from build123d import *

# Parameters (mm, degrees)
SKETCH_1_R          = 1.7
SKETCH_1_R_2        = 4
EXTRUDE_1_DEPTH     = 2
SKETCH_2_R          = 1.5
SKETCH_2_R_2        = 1.7
SKETCH_2_R_3        = 1.65
CUT_EXTRUDE_2_DEPTH = 100.30986231


with BuildPart() as part:
    # Эскиз1 → Бобышка-Вытянуть1 (new body)
    with BuildSketch(Plane(origin=(0, 0, 0), x_dir=(1, 0, 0), z_dir=(0, 1, 0))):
        with BuildLine():
            Line((-11.994516295, 0.362737998), (-27.997650279, 0.362737998))
            ThreePointArc((-27.997650279, 0.362737998), (-19.670324553, 19.926824433), (0, 28))
            ThreePointArc((0, 28), (10.092907112, 26.117680334), (18.828808684, 20.72380186))
            Line((18.828808684, 20.72380186), (46.640586318, -4.544855106))
            add(Edge.make_bspline(
                [(73.991805315, -64.992405718), (82.088977067, -40.455490793), (46.640586318, -4.544855106)],
                knots=[0.235504237, 0.235504237, 0.235504237, 1.570796327, 1.570796327, 1.570796327], degree=2, weights=[1, 0.785281266, 1]))
            Line((73.991805315, -64.992405718), (67.937451343, -58.859103325))
            add(Edge.make_bspline(
                [(67.937451343, -58.859103325), (68.070075227, -1.227091326), (11.741792344, -2.475946799)],
                knots=[3.541017893, 3.541017893, 3.541017893, 5.906750707, 5.906750707, 5.906750707], degree=2, weights=[1, 0.378272966, 1]))
            ThreePointArc((11.741792344, -2.475946799), (-1.424956207, -11.915095459), (-11.994516295, 0.362737998))
        make_face()
        with Locations(Location((-6.322604321, 6.40505071, 0), (0, 0, 270))):
            Circle(SKETCH_1_R, mode=Mode.SUBTRACT)
        with Locations(Location((0, 0, 0), (0, 0, 270))):
            Circle(SKETCH_1_R_2, mode=Mode.SUBTRACT)
        with Locations(Location((8.708238788, 2.273010605, 0), (0, 0, 270))):
            Circle(SKETCH_1_R, mode=Mode.SUBTRACT)
        with Locations(Location((-2.385634467, -8.678061315, 0), (0, 0, 270))):
            Circle(SKETCH_1_R, mode=Mode.SUBTRACT)
    extrude(amount=EXTRUDE_1_DEPTH)

    # Эскиз2 → Вырез-Вытянуть2 (cut, through all)
    with BuildSketch(Plane(origin=(0, 2, 0), x_dir=(1, 0, 0), z_dir=(0, 1, 0))):
        with Locations(Location((-4.341204442, 24.620193825, 0), (0, 0, 270))):
            Circle(SKETCH_2_R)
        with Locations(Location((-14.339410909, 20.478801107, 0), (0, 0, 90))):
            Circle(SKETCH_2_R)
        with Locations(Location((58.334133011, -29.525755439, 0), (0, 0, 270))):
            Circle(SKETCH_2_R_2)
        with Locations(Location((70.257880668, -52.24397848, 0), (0, 0, 270))):
            Circle(SKETCH_2_R_2)
        with Locations(Location((41.483595962, -12.455488374, 0), (0, 0, 270))):
            Circle(SKETCH_2_R_3)
    extrude(amount=-CUT_EXTRUDE_2_DEPTH, mode=Mode.SUBTRACT)


solid = part.part
Can you work these out from the model? Positions are in its coordinate system, mm. Round coordinates to 2 decimals unless told otherwise and drop trailing zeros. Order: outer loops, then holes, each group sorted by start corner. A loop starts at its lowest first (then second) coordinate and runs counter-clockwise, first axis right, second up. Notation, with made-up numbers: (-2, 1) - (7, 1) arc R12 ccw to (7, 20) - close; hole circle Ø8 at (41.5, 84). An arc over 180 degrees is marked (long way). Answer in a Markdown table with one row per item.
(1) For P1, Ø1, axis at y = 0.5, z = 8, coming from the -X side; P2, Ø1, axis at y = 0.5, z = 32.5, coming from the -X side, each with a flat end and sliding along its axis, tell me the tip position at first contact or that it passes through.
From the geometry:
| item | result |
|---|---|
| P1 | stops at x = -9.37 |
| P2 | stops at x = 55.87 |
(2) Suppose I cut it at C-C, the plane y = 1.2. Count the separate pieces of the cut face and the enclosed holes in it, plus the area to 3 significant figures.
From the geometry:
| item | result |
|---|---|
| separate pieces | 1 |
| enclosed holes | 9 |
| area | 2,280 mm2 |
(3) Please list where these lines run through material, in increasing order: L1, parallel to Z at x = 2, y = 0.25; L2, parallel to Z at x = -15.5, y = 0.15; L3, parallel to X at y = 0.8, z = 29. Write a range as from..to.
From the geometry:
| item | result |
|---|---|
| L1 | z = -27.93..-3.46, 3.46..11.83 |
| L2 | z = -23.32..-21.43, -19.53..-0.36 |
| L3 | x = 53.46..56.72, 59.95..65.6 |
(4) If we mould it in two halves opening along X, with no side actions, what happens to faces 1 (the face through (32.54, 0.986, -8.266)), 2 (the face through (19, 0, 1)), 3 (the face through (7.05, 0.99, -2.64)), 4 (the face through (71.01, 0.99, 61.97))? For each: released by +X, released by -X, zero draft, split by the parting line, or undercut.
From the geometry:
| item | result |
|---|---|
| face 1 | released by +X |
| face 2 | zero draft |
| face 3 | undercut |
| face 4 | released by -X |
(5) Suppose I cut it at D-D, the plane z = -13. Please give me the cut outline in (x, y), plus the area to 3 significant figures.
From the geometry:
| item | result |
|---|---|
| outline | (-24.8, 0) - (27.33, 0) - (27.33, 2) - (-24.8, 2) - close |
| area | 104 mm2 |
(6) Suppose I cut it at A-A, the plane x = 1.5. Please give me the cut outline in (y, z).
From the geometry:
| item | result |
|---|---|
| outline | (0, -27.96) - (2, -27.96) - (2, -3.71) - (0, -3.71) - close; (0, 3.71) - (2, 3.71) - (2, 11.91) - (0, 11.91) - close |
(7) Suppose I cut it at B-B, the plane x = -19.5. Please give me the cut outline in (y, z), plus the area to 3 significant figures.
From the geometry:
| item | result |
|---|---|
| outline | (0, -20.09) - (2, -20.09) - (2, -0.36) - (0, -0.36) - close |
| area | 39.5 mm2 |
